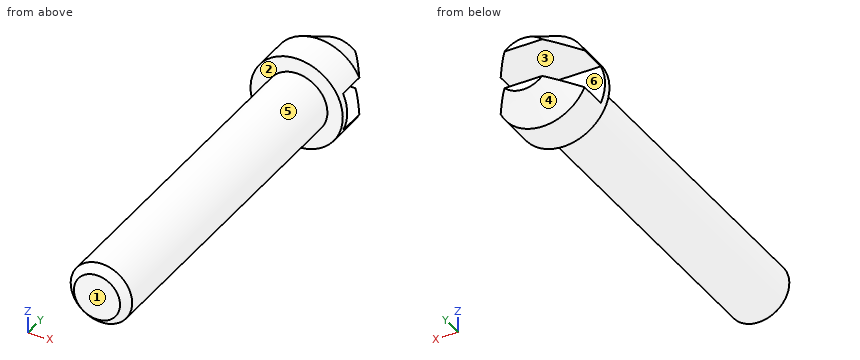
```python
from build123d import *

# Parameters (mm, degrees)
SKIZZE2_W                       = 14
SKIZZE2_H                       = 5
SCHNITT_LINEAR_AUSTRAGEN1_DEPTH = 8
FASE1_SIZE                      = 1


with BuildPart() as part:
    # Skizze1 → Rotation1 (revolve)
    with BuildSketch(Plane.XY, mode=Mode.PRIVATE) as rotation1_sk:
        Polygon((0, 0), (0, 54), (-3.5, 54), (-6, 49.669872981), (-6, 45), (-4, 45), (-4, 0), align=None)
    revolve(rotation1_sk.sketch.rotate(Axis((0, 0, 0), (0, -1, 0)), 270), axis=Axis((0, 0, 0), (0, -1, 0)))

    # Skizze2 → Schnitt-Linear austragen1 (cut)
    with BuildSketch(Plane(origin=(0, 54, 0), x_dir=(1, 0, 0), z_dir=(0, 1, 0))):
        Rectangle(SKIZZE2_W, SKIZZE2_H)
    extrude(amount=-SCHNITT_LINEAR_AUSTRAGEN1_DEPTH, mode=Mode.SUBTRACT)

    # Fase1
    fase1_edges = [part.edges().sort_by_distance(p)[0] for p in [
        (0, 0, -4),
    ]]
    chamfer(fase1_edges, length=FASE1_SIZE)


solid = part.part
```
The listing builds one solid part. Answer for the finished solid, in the listing's coordinates (mm). Face numbers are marked on the shaded views. A direction names the side the tool comes from. Give positions to 0.01 mm unless a question says otherwise; leave off trailing zeros. Order: outer loops, then holes, each group sorted by start corner. A loop starts at its lowest first (then second) coordinate and runs counter-clockwise, first axis right, second up. Notation, with made-up numbers: (67, 3) -> (72, 3) arc R22 ccw to (72, 22) -> close; hole circle Ø2 at (79, -23.75). An arc over 180 degrees is marked (long way). One line per item, written item: value.
1) Find section A-A, the plane x = 0. Determine the outline of the cut face in (y, z).
Reported:
outline: (0, -3) -> (1, -4) -> (45, -4) -> (45, -6) -> (49.67, -6) -> (54, -3.5) -> (54, -2.5) -> (46, -2.5) -> (46, 2.5) -> (54, 2.5) -> (54, 3.5) -> (49.67, 6) -> (45, 6) -> (45, 4) -> (1, 4) -> (0, 3) -> close
2) Find section B-B, the plane z = 0. Determine the outline of the cut face in (x, y), plus the area to 3 significant figures.
Reported:
outline: (-6, 45) -> (-4, 45) -> (-4, 1) -> (-3, 0) -> (3, 0) -> (4, 1) -> (4, 45) -> (6, 45) -> (6, 46) -> (-6, 46) -> close
area: 371 mm^2
3) Find the intervals of material crossed by line 1 (X direction, y = 27, z = -0.25); line 2 (Y direction, x = -4.25, z = -2.25); line 3 (Y direction, x = -1.25, z = -0.75), in increasing order.
Reported:
line 1: x = -3.99 to 3.99
line 2: y = 45 to 46
line 3: y = 0 to 46
4) Determine the mould class of the marked faces 4, 5 and 6 for opening direction Z: pulls with the +Z half, pulls with the -Z half, needs draft (parallel to the pull), parting line crosses it, or undercut.
Reported:
face 4: pulls with the -Z half
face 5: parting line crosses it
face 6: undercut
5) A tool of negligible diameter and unlimited length cuts with its end or side. For the marked faces 1, 2 and 3, from which of +Z, -Z, +X, -X, +Y, -Y can it reach the whole face along a straight path? Write none if from no direction.
Reported:
face 1: +Z, -Z, +X, -X, -Y
face 2: -Y
face 3: +X, -X, +Y
6) Flat-ended cylindrical pins translate along their axes: P1, Ø6, axis at x = -2, y = 11.5, coming from the +Z side; P2, Ø6.5, axis at x = -2, y = 49, coming from the -Z side; P3, Ø1.5, axis at x = 4, y = 37, coming from the +Z side; P4, Ø2, axis at x = 2.5, z = 4.5, coming from the -Y side. Find the tip coordinate at first contact, or state that the pin passes through.
Reported:
P1: stops at z = 4
P2: stops at z = -6
P3: stops at z = 2.33
P4: stops at y = 45
7) Find section C-C, the plane y = 37. Determine the outline of the cut face in (x, z).
Reported:
outline: circle Ø8 at (0, 0)
